```python
from build123d import *

# Parameters (mm, degrees)
F2_R     = 10.2989039919
F3_DEPTH = 3.175


# Not quite as in the source:
# - a length typed as a fraction of an inch, garbled in the dataset ("3 / 203.2 mm" for 3/8 in), is restored


with BuildPart() as f1:
    # F0 (on Front) → F1 (revolve)
    with BuildSketch(Plane.XZ):
        Polygon((0, 76.2), (0, 0), (3.175, 2.5115670547), (3.175, 70.6755), (9.525, 70.6755), (9.525, 71.4375), (4.7625, 73.025), (4.7625, 76.2), align=None)
    revolve(axis=Axis((0, 0, 38.1), (0, 0, 1)))

    # F2 (on face) → F3 (cut)
    with BuildSketch(Plane.XY.offset(76.2)):
        Circle(F2_R)
        Polygon((-4.7625, 0), (-2.38125, 4.1244459855), (2.38125, 4.1244459855), (4.7625, 0), (2.38125, -4.1244459855), (-2.38125, -4.1244459855), align=None, mode=Mode.SUBTRACT)
    extrude(amount=-F3_DEPTH, mode=Mode.SUBTRACT)


solid = f1.part
```
Here's how the part is built. I have some questions about the finished solid (model axes, mm). A direction names the side the tool comes from. Coordinates: 2 decimals unless noted, no trailing zeros. Order: outer loops, then holes, each group sorted by start corner. A loop starts at its lowest first (then second) coordinate and runs counter-clockwise, first axis right, second up.
Item 1: I'm going to push flat-ended pins straight in: pin 1 Ø2.5 at (x, z) = (0.5, 74.5) entering from +Y; pin 2 Ø2 at (x, z) = (-5.5, 33) entering from +Y; pin 3 Ø2 at (x, z) = (1, 66) entering from +Y (3 decimals); pin 4 Ø2.5 at (x, y) = (4, 2) entering from +Z. Where does each tip first touch, or does it pass through?
Response values:
pin 1: stops at y = 4.12
pin 2: passes through
pin 3: stops at y = 3.175
pin 4: stops at z = 76.2
Item 2: I need wall thicknesses on probe 1 along Z at (x, y) = (-1.75, 4); probe 2 along Z at (x, y) = (-1, 5.25); probe 3 along X at (y, z) = (1, 30). Which ranges of each line are inside material? Lowest first, please.
Response values:
probe 1: z = 70.68 to 76.2
probe 2: z = 70.68 to 72.83
probe 3: x = -3.01 to 3.01
Item 3: If we section it at A-A, the plane z = 62.5: List the corners of the cut face in (x, y) for me (3 decimals).
Response values:
outline: circle Ø6.35 at (0, 0)
Item 4: Which directions (+Z, -Z, +X, -X, +Y, -Y) give clear straight access to the entire face, cutting with the end or side of a thin tool? Please do faces 1 (the face through (4, -2, 73.025)), 2 (the face through (-3.555, -2.091, 74.635)), 3 (the face through (-4, 2, 73.025)).
Response values:
face 1: +Z, +X, -Y
face 2: +Z, -X, -Y
face 3: +Z, -X, +Y
